The model under review builds one solid part; all positions refer to its coordinate system, in mm. A direction names the side the tool comes from. Give positions to 0.01 mm unless a question says otherwise; leave off trailing zeros. Loops run counter-clockwise (first coordinate to the right, second up) from the corner with the lowest first, then second, coordinate; pieces in that order, holes last. Notation, with made-up numbers: M 46.5,-23 L 102.5,-23 A20 ccw 102.5,-5 Z; hole C -5.75,46 d2. An arc over 180 degrees is marked long. Return JSON: item names as keys, results as strings.
```python
from build123d import *

# Parameters (mm, degrees)
F0_R      = 53
F0_R_2    = 38.875
F1_DEPTH  = 2
F2_W      = 15.987269
F2_H      = 100
F3_DEPTH  = 25
F4_R      = 41.175
F5_DEPTH  = 1.3
F6_R      = 42.86
F6_R_2    = 38.875
F7_DEPTH  = 6.25
F8_R      = 1.37
F9_DEPTH  = 25
F10_W     = 16.146997
F10_H     = 16.86
F11_DEPTH = 0.65


with BuildPart() as f1:
    # F0 (on Front) → F1 (new body)
    with BuildSketch(Plane.XZ):
        Circle(F0_R)
        Circle(F0_R_2, mode=Mode.SUBTRACT)
    extrude(amount=F1_DEPTH)

    # F2 (on face) → F3 (cut)
    with BuildSketch(Plane.XZ.offset(2)):
        with Locations((53.868634, 20.202986)):
            Rectangle(F2_W, F2_H)
    extrude(amount=-F3_DEPTH, mode=Mode.SUBTRACT)

    # F4 (on face) → F5 (cut)
    with BuildSketch(Plane.XZ.offset(2)):
        Circle(F4_R)
    extrude(amount=-F5_DEPTH, mode=Mode.SUBTRACT)

    # F6 (on face) → F7 (join)
    with BuildSketch(Plane(origin=(0, 0, 0), x_dir=(-1, 0, 0), z_dir=(0, 1, 0))):
        Circle(F6_R)
        Circle(F6_R_2, mode=Mode.SUBTRACT)
    extrude(amount=F7_DEPTH)

    # F8 (on face) → F9 (cut)
    with BuildSketch(Plane.XZ.offset(2)):
        with Locations((0, 47)):
            Circle(F8_R)
        with Locations((0, -47)):
            Circle(F8_R)
        with Locations((40.264472, 24.244016)):
            Circle(F8_R)
        with Locations((-40.264472, 24.244016)):
            Circle(F8_R)
        with Locations((-40.264472, -24.244016)):
            Circle(F8_R)
        with Locations((40.264472, -24.244016)):
            Circle(F8_R)
    extrude(amount=-F9_DEPTH, mode=Mode.SUBTRACT)

    # F10 (on face) → F11 (cut)
    with BuildSketch(Plane.XZ.offset(2)):
        with Locations((43.073498, 0)):
            Rectangle(F10_W, F10_H)
    extrude(amount=-F11_DEPTH, mode=Mode.SUBTRACT)


solid = f1.part
```
1) Insertion check: pin 1 (2 mm diameter, centred on x = 0, z = 47, fed in from +Y); pin 2 (1 mm diameter, centred on y = 2.5, z = -9, fed in from +X); pin 3 (6 mm diameter, centred on x = 43, z = -3, fed in from -Y); pin 4 (4 mm diameter, centred on x = -24.5, y = 3.5, fed in from +Z). Each pin has a flat end and moves straight along its axis. Give the tip position at first contact, or say it passes through.
From the geometry:
{"pin 1": "through", "pin 2": "x = 42.01", "pin 3": "y = -1.35", "pin 4": "z = 36.48"}
2) Consider section A-A on x = 0. Write out the cut boundary in (y, z) (3 decimals).
From the geometry:
{"outline": "M -2,-53 L 0,-53 L 0,-48.37 L -2,-48.37 Z; M -2,-45.63 L 0,-45.63 L 0,-42.86 L 6.25,-42.86 L 6.25,-38.875 L -0.7,-38.875 L -0.7,-41.175 L -2,-41.175 Z; M -2,41.175 L -0.7,41.175 L -0.7,38.875 L 6.25,38.875 L 6.25,42.86 L 0,42.86 L 0,45.63 L -2,45.63 Z; M -2,48.37 L 0,48.37 L 0,53 L -2,53 Z"}
3) Wall thickness on L1, parallel to Z at x = 0, y = -1.35 (3 decimals); L2, parallel to X at y = -0.2, z = 0 (3 decimals); L3, parallel to Y at x = -41.5, z = 27: over which ranges is each line inside the solid? List them lowest first. Write a range as from..to.
From the geometry:
{"L1": "-53..-48.37, -45.63..-41.175, 41.175..45.63, 48.37..53", "L2": "-53..-38.875, 38.875..45.875", "L3": "-2..0"}
4) Consider section D-D on y = 3. Write out the cut boundary in (x, z) (3 decimals), then the cut area to 3 significant figures.
From the geometry:
{"outline": "C 0,0 d85.72; hole C 0,0 d77.75", "area": "1,020 mm²"}
5) Tool access review of faces 4 (the face through (30, -0.7, 25)), 5 (the face through (43, -1.35, 0)), 6 (the face through (34.01, 3.08, -26.08)): name each direction out of +Z, -Z, +X, -X, +Y, -Y from which nothing blocks a thin tool from reaching the whole face with its end or side.
From the geometry:
{"face 4": "-Y", "face 5": "+X, -Y", "face 6": "+Y"}
6) Consider section C-C on x = -23. Write out the cut boundary in (y, z).
From the geometry:
{"outline": "M -2,-47.75 L 0,-47.75 L 0,-36.17 L 6.25,-36.17 L 6.25,-31.34 L -0.7,-31.34 L -0.7,-34.15 L -2,-34.15 Z; M -2,34.15 L -0.7,34.15 L -0.7,31.34 L 6.25,31.34 L 6.25,36.17 L 0,36.17 L 0,47.75 L -2,47.75 Z"}
7) Consider section B-B on z = 0. Write out the cut boundary in (x, y) (3 decimals).
From the geometry:
{"outline": "M -53,-2 L -41.175,-2 L -41.175,-0.7 L -38.875,-0.7 L -38.875,6.25 L -42.86,6.25 L -42.86,0 L -53,0 Z; M 38.875,-0.7 L 41.175,-0.7 L 41.175,-1.35 L 45.875,-1.35 L 45.875,0 L 42.86,0 L 42.86,6.25 L 38.875,6.25 Z"}
8) The part is to be moulded in two halves that separate along X. For faces 1 (the face through (-52.964, -0.986, 1.941)), 2 (the face through (-0.297, -1.014, -48.337)), 3 (the face through (-9, 6.25, -38)), say which applies: released by +X, released by -X, zero draft, split by the parting line, or undercut.
From the geometry:
{"face 1": "split by the parting line", "face 2": "undercut", "face 3": "zero draft"}
